Can you work these out from the model? Positions are in its coordinate system, mm. Face numbers are marked on the shaded views. Coordinates: 2 decimals unless noted, no trailing zeros. Order: outer loops, then holes, each group sorted by start corner. A loop starts at its lowest first (then second) coordinate and runs counter-clockwise, first axis right, second up. Notation, with made-up numbers: (-31, 26) -> (16, 26) arc R7 ccw to (16, 39) -> close; hole circle Ø1 at (61.25, 63.5). An arc over 180 degrees is marked (long way). Answer in a Markdown table with one row per item.
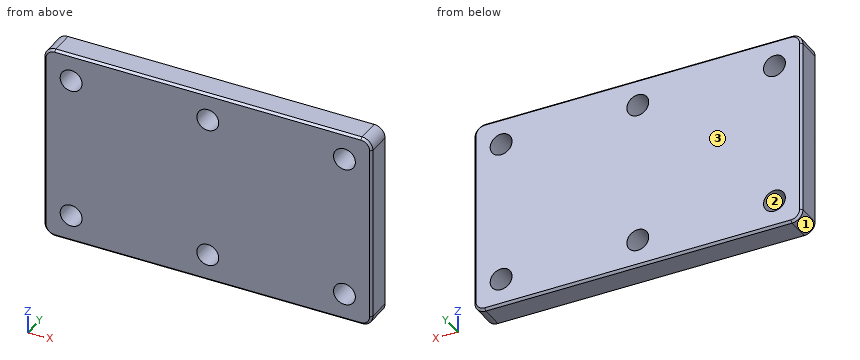
```python
from build123d import *

# Parameters (mm, degrees)
SKETCH1_R           = 10
BOSS_EXTRUDE1_DEPTH = 12.5
CHAMFER1_SIZE       = 2


with BuildPart() as part:
    # Sketch1 → Boss-Extrude1 (new, symmetric)
    with BuildSketch(Plane(origin=(0, 0, 0), x_dir=(1, 0, 0), z_dir=(0, 1, 0))):
        with BuildLine():
            Line((10, 0), (290, 0))
            ThreePointArc((290, 0), (297.071067812, -2.928932188), (300, -10))
            Line((300, -10), (300, -170))
            ThreePointArc((300, -170), (297.071067812, -177.071067812), (290, -180))
            Line((290, -180), (10, -180))
            ThreePointArc((10, -180), (2.928932188, -177.071067812), (0, -170))
            Line((0, -170), (0, -10))
            ThreePointArc((0, -10), (2.928932188, -2.928932188), (10, 0))
        make_face()
        with Locations(Location((25, -25, 0), (0, 0, 270))):
            Circle(SKETCH1_R, mode=Mode.SUBTRACT)
        with Locations(Location((25, -155, 0), (0, 0, 270))):
            Circle(SKETCH1_R, mode=Mode.SUBTRACT)
        with Locations(Location((275, -25, 0), (0, 0, 270))):
            Circle(SKETCH1_R, mode=Mode.SUBTRACT)
        with Locations(Location((275, -155, 0), (0, 0, 270))):
            Circle(SKETCH1_R, mode=Mode.SUBTRACT)
        with Locations(Location((150, -25, 0), (0, 0, 270))):
            Circle(SKETCH1_R, mode=Mode.SUBTRACT)
        with Locations(Location((150, -155, 0), (0, 0, 270))):
            Circle(SKETCH1_R, mode=Mode.SUBTRACT)
    extrude(amount=BOSS_EXTRUDE1_DEPTH, both=True)

    # Chamfer1
    chamfer1_edges = [part.edges().sort_by_distance(p)[0] for p in [
        (150, -12.5, 0),
        (297.071067812, -12.5, 2.928932188),
        (300, -12.5, 90),
        (297.071067812, -12.5, 177.071067812),
        (297.071067812, 12.5, 2.928932188),
        (150, 12.5, 0),
        (2.928932188, 12.5, 2.928932188),
        (0, 12.5, 90),
        (2.928932188, 12.5, 177.071067812),
        (150, 12.5, 180),
        (297.071067812, 12.5, 177.071067812),
        (150, -12.5, 180),
        (300, 12.5, 90),
        (2.928932188, -12.5, 177.071067812),
        (0, -12.5, 90),
        (2.928932188, -12.5, 2.928932188),
    ]]
    chamfer(chamfer1_edges, length=CHAMFER1_SIZE)


solid = part.part
```
(1) Suppose I cut it at B-B (y = 4.25). Please give me the cut outline in (x, z).
Response values:
| item | result |
|---|---|
| outline | (0, 10) arc R10 ccw to (10, 0) -> (290, 0) arc R10 ccw to (300, 10) -> (300, 170) arc R10 ccw to (290, 180) -> (10, 180) arc R10 ccw to (0, 170) -> close; hole circle Ø20 at (25, 25); hole circle Ø20 at (25, 155); hole circle Ø20 at (150, 25); hole circle Ø20 at (150, 155); hole circle Ø20 at (275, 25); hole circle Ø20 at (275, 155) |
(2) Will this pin go through, and if not, where does the flat tip stop? pin 1 Ø12 at (x, z) = (150, 25) entering from -Y.
Response values:
| item | result |
|---|---|
| pin 1 | through |
(3) Suppose I cut it at C-C (x = 150). Please give me the cut outline in (y, z).
Response values:
| item | result |
|---|---|
| outline | (-12.5, 2) -> (-10.5, 0) -> (10.5, 0) -> (12.5, 2) -> (12.5, 15) -> (-12.5, 15) -> close; (-12.5, 35) -> (12.5, 35) -> (12.5, 145) -> (-12.5, 145) -> close; (-12.5, 165) -> (12.5, 165) -> (12.5, 178) -> (10.5, 180) -> (-10.5, 180) -> (-12.5, 178) -> close |
(4) We'd pull the mould along X, two halves only. Please class the marked faces 1, 2 and 3: +X half, -X half, draft (parallel to the pull), parting line (faces both ways), or undercut.
Response values:
| item | result |
|---|---|
| face 1 | -X half |
| face 2 | undercut |
| face 3 | draft |
(5) I need wall thicknesses on line 1 (X direction, y = 0.75, z = 155); line 2 (X direction, y = -0.75, z = 152); line 3 (X direction, y = 11.75, z = 107). Which ranges of each line are inside material? Lowest first, please. Write a range as [from, to].
Response values:
| item | result |
|---|---|
| line 1 | [0, 15], [35, 140], [160, 265], [285, 300] |
| line 2 | [0, 15.46], [34.54, 140.46], [159.54, 265.46], [284.54, 300] |
| line 3 | [1.25, 298.75] |
(6) Suppose I cut it at D-D (z = 160). Please give me the cut outline in (x, y), and give its area (3 significant figures).
Response values:
| item | result |
|---|---|
| outline | (0, -10.5) -> (2, -12.5) -> (16.34, -12.5) -> (16.34, 12.5) -> (2, 12.5) -> (0, 10.5) -> close; (33.66, -12.5) -> (141.34, -12.5) -> (141.34, 12.5) -> (33.66, 12.5) -> close; (158.66, -12.5) -> (266.34, -12.5) -> (266.34, 12.5) -> (158.66, 12.5) -> close; (283.66, -12.5) -> (298, -12.5) -> (300, -10.5) -> (300, 10.5) -> (298, 12.5) -> (283.66, 12.5) -> close |
| area | 6,190 mm2 |
(7) Suppose I cut it at A-A (z = 25). Please give me the cut outline in (x, y).
Response values:
| item | result |
|---|---|
| outline | (0, -10.5) -> (2, -12.5) -> (15, -12.5) -> (15, 12.5) -> (2, 12.5) -> (0, 10.5) -> close; (35, -12.5) -> (140, -12.5) -> (140, 12.5) -> (35, 12.5) -> close; (160, -12.5) -> (265, -12.5) -> (265, 12.5) -> (160, 12.5) -> close; (285, -12.5) -> (298, -12.5) -> (300, -10.5) -> (300, 10.5) -> (298, 12.5) -> (285, 12.5) -> close |
